The drawing under review shows one solid part. Ordinate dimensions are in mm from its lowest x, y, z. Coordinates: 2 decimals unless noted, no trailing zeros. Write each loop counter-clockwise with the first axis right and the second up, starting at its lowest first coordinate (ties: lowest second). Pieces come first, ordered by that corner, then holes. Notation, with made-up numbers: (-10.75, -15.75) -> (-1.75, -15.75) arc R18 ccw to (-1.75, 19.25) -> close; hole circle Ø3 at (-24.75, 21). An arc over 180 degrees is marked (long way). One line per question, with ' | ' between items. Start each with the question number.
Q1. Add section A-A on z = 2.35. State the section outline as (x, y) points (3 decimals), and give its area (3 significant figures).
Q2. For P1, Ø1.5, axis at y = 35, z = 3, coming from the -X side; P2, Ø0.8, axis at x = 18.5, y = 1, coming from the +Z side; P3, Ø0.5, axis at y = 2, z = 2.5, coming from the -X side (3 decimals); P4, Ø0.8, axis at y = 1.5, z = 2, coming from the +X side (3 decimals), all flat-tipped, find the tip position at first contact; note any pin that passes through.
Q3. Add section B-B on x = 3. State the section outline as (y, z) points, and give its area (3 significant figures).
Q4. Add section C-C on z = 4.4. State the section outline as (x, y) points.
Q5. Wall thickness on probe 1 along Y at (x, z) = (13.5, 3.35); probe 2 along X at (y, z) = (13, 4.6); probe 3 along X at (y, z) = (23, 0.75): over which ranges is each line inside the solid? List them lowest first.
Q6. Draft analysis for pull direction Z (two halves, no side actions). For the marked faces 1, 2 and 3, state which applies: pulls with the +Z half, pulls with the -Z half, needs draft (parallel to the pull), parting line crosses it, or undercut.
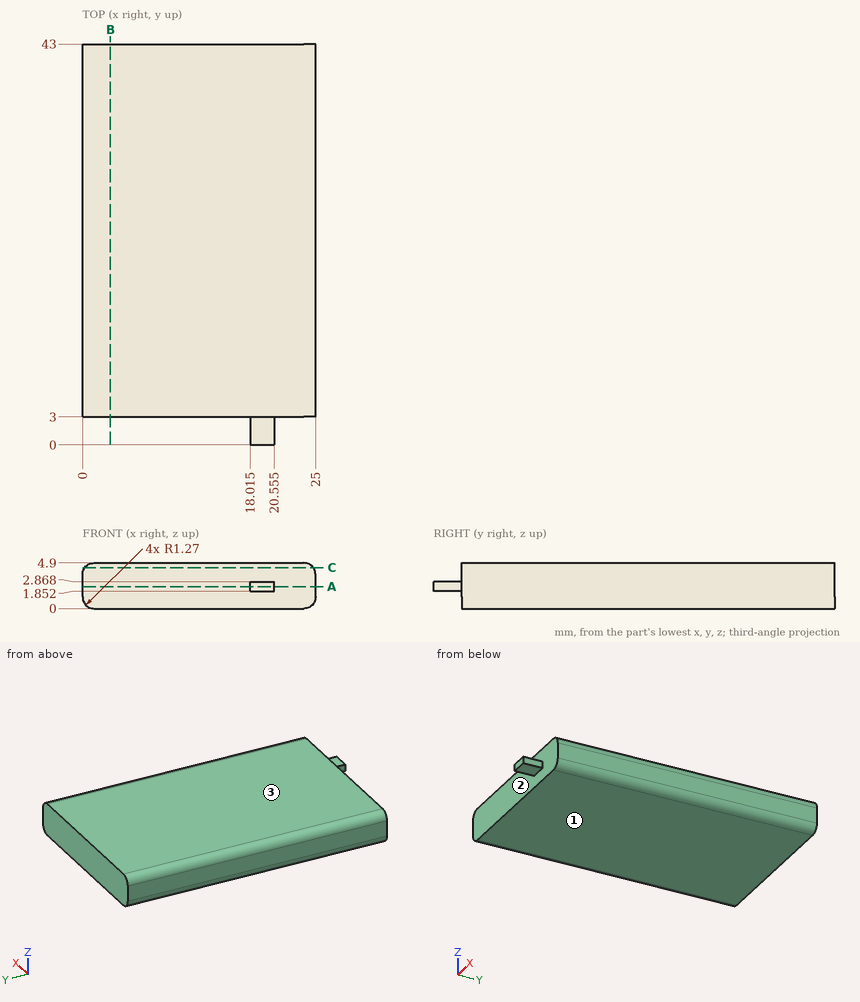
Output values:
1) outline: (0, 3) -> (18.015, 3) -> (18.015, 0) -> (20.555, 0) -> (20.555, 3) -> (25, 3) -> (25, 43) -> (0, 43) -> close | area: 1,010 mm2
2) P1: stops at x = 0 | P2: stops at z = 2.87 | P3: stops at x = 18.015 | P4: stops at x = 20.555
3) outline: (3, 0) -> (43, 0) -> (43, 4.9) -> (3, 4.9) -> close | area: 196 mm2
4) outline: (0.26, 3) -> (24.74, 3) -> (24.74, 43) -> (0.26, 43) -> close
5) probe 1: y = 3 to 43 | probe 2: x = 0.45 to 24.55 | probe 3: x = 0.11 to 24.89
6) face 1: pulls with the -Z half | face 2: needs draft | face 3: pulls with the +Z half
